Read the model definition and answer for the solid it produces. Units are mm, in the model's axes. Face numbers are marked on the shaded views. A direction names the side the tool comes from. Coordinates: 2 decimals unless noted, no trailing zeros. Loops run counter-clockwise (first coordinate to the right, second up) from the corner with the lowest first, then second, coordinate; pieces in that order, holes last. Notation, with made-up numbers: M -32.5,-9 L -11.5,-9 A22 cw -11.5,2 Z; hole C 25,61 d3. An arc over 180 degrees is marked long. One line per item, written item: value. Start each with the question number.
```python
from build123d import *

# Parameters (mm, degrees)
EXTRUDE_1_DEPTH            = 78
SKETCH_3_R                 = 22.5
EXTRUDE_2_DEPTH            = 3.5
EXTRUDE_START              = 3.5
SKETCH_4_R                 = 22.5
EXTRUDE_3_DEPTH            = 3.5
SKETCH_5_W                 = 1.5
SKETCH_5_H                 = 36.764720589
CUT_EXTRUDE_1_DEPTH        = 97.598395432
SKETCH_6_R                 = 14
CUT_EXTRUDE_2_DEPTH        = 97.598395432
EXTRUDE_4_DEPTH            = 71
EXTRUDE_5_DEPTH            = 15
FILLET_1_R                 = 7
EXTRUDE_6_DEPTH            = 70
SKETCH_10_W                = 35
SKETCH_10_H                = 23.870791075
CUT_EXTRUDE_3_DEPTH        = 3.5
SKETCH_11_R                = 27
EXTRUDE_7_DEPTH            = 16
EXTRUDE_START_2            = 16
SKETCH_12_R                = 27
EXTRUDE_8_DEPTH            = 16
EXTRUDE_START_3            = 68
SKETCH_13_R                = 27
EXTRUDE_9_DEPTH            = 68
SKETCH_16_R                = 15
CUT_EXTRUDE_4_DEPTH        = 163.687584038
FILLET_2_R                 = 0.5
HOLE_WIZARD_5_8_18_1_D     = 14.68374
HOLE_WIZARD_5_8_18_1_DEPTH = 38.7985
HOLE_WIZARD_5_8_18_1_TIP   = 4.411440553


with BuildPart() as part:
    # 草图1 → 拉伸1 (new body)
    with BuildSketch(Plane(origin=(0, 0, 0), x_dir=(1, 0, 0), z_dir=(0, 1, 0))):
        with BuildLine():
            Line((-10, 20.155644371), (-10, 40))
            Line((-10, 40), (10, 40))
            Line((10, 40), (10, 20.155644371))
            ThreePointArc((10, 20.155644371), (0, -22.5), (-10, 20.155644371))
        make_face()
    extrude(amount=EXTRUDE_1_DEPTH)

    # 草图3 → 拉伸2 (add)
    with BuildSketch(Plane(origin=(0, 78, 0), x_dir=(1, 0, 0), z_dir=(0, 1, 0))):
        with Locations(Location((0, 0, 0), (0, 0, 63.612200039))):
            Circle(SKETCH_3_R)
    extrude(amount=EXTRUDE_2_DEPTH)

    # 草图4 → 拉伸3 (add)
    with BuildSketch(Plane.XZ.offset(EXTRUDE_START)):
        with Locations(Location((0, 0, 0), (0, 0, 270))):
            Circle(SKETCH_4_R)
    extrude(amount=-EXTRUDE_3_DEPTH)

    # 草图5 → 切除-拉伸1 (cut, through all)
    with BuildSketch(Plane(origin=(0, 81.5, 0), x_dir=(1, 0, 0), z_dir=(0, 1, 0))):
        with Locations((0, 23.144665006)):
            Rectangle(SKETCH_5_W, SKETCH_5_H)
    extrude(amount=-CUT_EXTRUDE_1_DEPTH, mode=Mode.SUBTRACT)

    # 草图6 → 切除-拉伸2 (cut, through all)
    with BuildSketch(Plane(origin=(0, 81.5, 0), x_dir=(1, 0, 0), z_dir=(0, 1, 0))):
        Circle(SKETCH_6_R)
    extrude(amount=-CUT_EXTRUDE_2_DEPTH, mode=Mode.SUBTRACT)

    # 草图7 → 拉伸4 (add)
    with BuildSketch(Plane.XY.offset(10)):
        Polygon((-17.5, 78), (17.5, 78), (17.5, 71.5), (0, 58), (-17.5, 71.5), align=None)
        Polygon((-17.5, 6.5), (0, 20), (17.5, 6.5), (17.5, 0), (-17.5, 0), align=None)
    extrude(amount=EXTRUDE_4_DEPTH)

    # 草图8 → 拉伸5 (add)
    with BuildSketch(Plane(origin=(0, 81.5, 0), x_dir=(1, 0, 0), z_dir=(0, 1, 0))):
        Polygon((-43, -113), (43, -113), (17.5, -81), (0, -59.039215686), (-17.5, -81), align=None)
    extrude(amount=-EXTRUDE_5_DEPTH)

    # 圆角1
    fillet_1_edges = [part.edges().sort_by_distance(p)[0] for p in [
        (-43, 74, 113),
        (0, 79.75, 59.039215686),
        (43, 74, 113),
    ]]
    fillet(fillet_1_edges, radius=FILLET_1_R)

    # 草图9 → 拉伸6 (add)
    with BuildSketch(Plane.XZ.offset(-66.5)):
        Polygon((-25.881035827, 113), (26.118964173, 113), (26.118964173, 91.81595504), (0, 58.326677723), (-25.881035827, 91.517378293), align=None)
    extrude(amount=EXTRUDE_6_DEPTH)

    # 草图10 → 切除-拉伸3 (cut)
    with BuildSketch(Plane.XZ.offset(3.5)):
        with Locations((0, 69.064604463)):
            Rectangle(SKETCH_10_W, SKETCH_10_H)
    extrude(amount=-CUT_EXTRUDE_3_DEPTH, mode=Mode.SUBTRACT)

    # 草图11 → 拉伸7 (add)
    with BuildSketch(Plane(origin=(26.118964173, 0, 0), x_dir=(0, 0, -1), z_dir=(1, 0, 0))):
        with Locations(Location((-76.5, 39, 0), (0, 0, 235.440790003))):
            Circle(SKETCH_11_R)
    extrude(amount=EXTRUDE_7_DEPTH)

    # 草图12 → 拉伸8 (add)
    with BuildSketch(Plane.ZY.offset(25.881035827).offset(EXTRUDE_START_2)):
        with Locations(Location((76.5, 39, 0), (0, 0, 304.559209997))):
            Circle(SKETCH_12_R)
    extrude(amount=-EXTRUDE_8_DEPTH)

    # 草图13 → 拉伸9 (add)
    with BuildSketch(Plane.ZY.offset(-26.118964173).offset(EXTRUDE_START_3)):
        with Locations((76.5, 39)):
            Circle(SKETCH_13_R)
    extrude(amount=-EXTRUDE_9_DEPTH)

    # 草图16 → 切除-拉伸4 (cut, through all)
    with BuildSketch(Plane(origin=(42.118964173, 0, 0), x_dir=(0, 0, -1), z_dir=(1, 0, 0))):
        with Locations((-76.5, 39)):
            Circle(SKETCH_16_R)
    extrude(amount=-CUT_EXTRUDE_4_DEPTH, mode=Mode.SUBTRACT)

    # 圆角2
    fillet_2_edges = [part.edges().sort_by_distance(p)[0] for p in [
        (42.118964173, 61.235591317, 61.18404496),
        (-41.881035827, 51.559243885, 52.598841178),
        (-41.881035827, 39, 91.5),
        (42.118964173, 39, 91.5),
    ]]
    fillet(fillet_2_edges, radius=FILLET_2_R)

    # 5/8-18 螺纹孔1
    with Locations(Plane(origin=(10, 0, 0), x_dir=(0, 0, -1), z_dir=(1, 0, 0))):
        with Locations((30.077822185, 63), (30.077822185, 15)):
            Hole(HOLE_WIZARD_5_8_18_1_D / 2, depth=HOLE_WIZARD_5_8_18_1_DEPTH)
            with Locations((0, 0, -(HOLE_WIZARD_5_8_18_1_DEPTH + HOLE_WIZARD_5_8_18_1_TIP / 2))):  # 118° drill point
                Cone(0, HOLE_WIZARD_5_8_18_1_D / 2, HOLE_WIZARD_5_8_18_1_TIP, mode=Mode.SUBTRACT)


solid = part.part
```
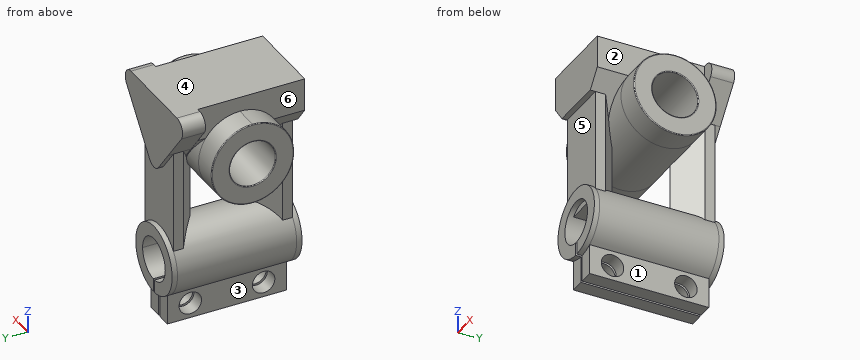
1) Consider line 1 along X through (y, z) = (24, -23.5); line 2 along Y through (x, z) = (15.5, 56.5); line 3 along Z through (x, y) = (-8.5, 14.5). Determine where each line is inside the solid, lowest interval first.
2) Section B-B (x = 31) is taken. Determine the outline of the cut face in (y, z), then the cut area to 3 significant figures.
3) A tool of negligible diameter and unlimited length cuts with its end or side. For the marked faces 1, 2 and 3, from which of +Z, -Z, +X, -X, +Y, -Y can it reach the whole face along a straight path? Write none if from no direction.
4) Section A-A (z = 29) is taken. Determine the outline of the cut face in (x, y).
5) For a pull along Z with two mould halves and no side action, classify the marked faces 4, 5 and 6 as released by +Z, released by -Z, zero draft, split by the parting line, or undercut.
6) Flat-ended cylindrical pins translate along their axes: pin 1 (10 mm diameter, centred on x = -19, y = 27, fed in from -Z); pin 2 (4.5 mm diameter, centred on x = -4.5, z = -30, fed in from +Y); pin 3 (7.5 mm diameter, centred on x = 28.5, z = 98, fed in from -Y); pin 4 (3 mm diameter, centred on y = 4, z = 59, fed in from -X). Find the tip coordinate at first contact, or state that the pin passes through.
7) Section C-C (y = 15) is taken. Count the separate pieces of the cut face and the enclosed holes in it, then the cut area to 3 significant figures.
Results found:
1. line 1: x = -10 to -0.75, 0.75 to 10
1. line 2: y = 0 to 8.04, 20.86 to 57.14, 69.96 to 78
1. line 3: z = -40 to -37.4, -22.75 to -11.12, 11.12 to 20.83, 65.15 to 113
2. outline: C 39,76.5 d54; M 66.5,97.94 L 81.5,97.94 L 81.5,112.53 L 66.5,112.53 Z; hole C 39,76.5 d30
2. area: 1,800 mm²
3. face 1: -Z, +X, +Y, -Y
3. face 2: +Z, +X
3. face 3: -Z, -X, +Y, -Y
4. outline: M -17.5,0 L 17.5,0 L 17.5,6.5 L 0,20 L -17.5,6.5 Z; M -17.5,71.5 L 0,58 L 17.5,71.5 L 17.5,78 L -17.5,78 Z
5. face 4: released by +Z
5. face 5: undercut
5. face 6: zero draft
6. pin 1: stops at z = -17.61
6. pin 2: stops at y = 78
6. pin 3: stops at y = -3.5
6. pin 4: stops at x = -17.5
7. separate pieces: 3
7. enclosed holes: 0
7. area: 4,940 mm²
